```python
from build123d import *

# Parameters (mm, degrees)
SKETCH_1_R                = 20
SKETCH_1_R_2              = 11
EXTRUDE_1_DEPTH           = 60
EXTRUDE_2_DEPTH           = 30
SKETCH_4_R                = 11
EXTRUDE_3_DEPTH           = 5
SKETCH_8_R                = 11
CUT_EXTRUDE_1_DEPTH       = 100
FILLET_4_R                = 20
EXTRUDE_START             = -30
SKETCH_18_R               = 35
EXTRUDE_4_DEPTH           = 5
EXTRUDE_START_2           = -25
SKETCH_19_R               = 35
EXTRUDE_5_DEPTH           = 5
FILLET_5_R                = 10
CUT_EXTRUDE_9_DEPTH       = 388.169213652
CUT_EXTRUDE_9_DEPTH_BACK  = 388.169213652
SKETCH_21_R               = 2.6
CUT_EXTRUDE_10_DEPTH      = 407.881000043
CUT_EXTRUDE_10_DEPTH_BACK = 407.881000043
SKETCH_22_W               = 65
SKETCH_22_H               = 431.087956996
MOVE_FACE_1_BY            = 0.1


with BuildPart() as part:
    # 草图1 → 凸台-拉伸1 (new body)
    with BuildSketch(Plane.XY):
        Circle(SKETCH_1_R)
        Circle(SKETCH_1_R_2, mode=Mode.SUBTRACT)
    extrude(amount=EXTRUDE_1_DEPTH)

    # 草图2 → 凸台-拉伸2 (add, symmetric)
    with BuildSketch(Plane.XY.offset(30)):
        with BuildLine():
            Line((-14.142135624, 14.142135624), (-90, -61.715728753))
            Line((-90, -61.715728753), (-90, -320))
            Line((-90, -320), (-50, -320))
            Line((-50, -320), (-50, -78.284271247))
            Line((-50, -78.284271247), (14.142135624, -14.142135624))
            ThreePointArc((14.142135624, -14.142135624), (-14.142135624, -14.142135624), (-14.142135624, 14.142135624))
        make_face()
    extrude(amount=EXTRUDE_2_DEPTH, both=True)

    # 草图4 → 凸台-拉伸3 (add)
    with BuildSketch(Plane.XY.offset(60)):
        with BuildLine():
            Line((-90, -290), (-50, -290))
            Line((-50, -290), (-50, -350))
            ThreePointArc((-50, -350), (-70, -370), (-90, -350))
            Line((-90, -350), (-90, -290))
        make_face()
        with Locations((-70, -350)):
            Circle(SKETCH_4_R, mode=Mode.SUBTRACT)
    extrude_3 = extrude(amount=EXTRUDE_3_DEPTH)

    # 镜向1: 凸台-拉伸3 across plane
    add(extrude_3.mirror(Plane.XY.offset(30)))

    # 草图8 → 切除-拉伸1 (cut)
    with BuildSketch(Plane.XY.offset(60)):
        with Locations((-35.355339059, -35.355339059)):
            Circle(SKETCH_8_R)
    extrude(amount=-CUT_EXTRUDE_1_DEPTH, mode=Mode.SUBTRACT)

    # 圆角4
    fillet_4_edges = [part.edges().sort_by_distance(p)[0] for p in [
        (-50, -78.284271247, 30),
        (-90, -61.715728753, 30),
    ]]
    fillet(fillet_4_edges, radius=FILLET_4_R)

    # 草图18 → 凸台-拉伸4 (add)
    with BuildSketch(Plane.XY.offset(60).offset(EXTRUDE_START)):
        with BuildLine():
            ThreePointArc((15.487252676, -12.654841151), (14.833346688, -13.415357842), (14.142135624, -14.142135624))
            Line((14.142135624, -14.142135624), (-44.142135624, -72.426406871))
            ThreePointArc((-44.142135624, -72.426406871), (-48.47759065, -78.914873848), (-50, -86.568542495))
            Line((-50, -86.568542495), (-50, -128.513280962))
            Line((-50, -128.513280962), (20.291868618, -128.513280962))
            ThreePointArc((20.291868618, -128.513280962), (62.790327113, -100.116718851), (52.818780552, -49.986369028))
            Line((52.818780552, -49.986369028), (15.487252676, -12.654841151))
        make_face()
        with Locations((20.291868618, -82.513280962)):
            Circle(SKETCH_18_R, mode=Mode.SUBTRACT)
    extrude(amount=EXTRUDE_4_DEPTH)

    # 草图19 → 凸台-拉伸5 (add)
    with BuildSketch(Plane(origin=(0, 0, 0), x_dir=(-1, 0, 0), z_dir=(0, 0, -1)).offset(EXTRUDE_START_2)):
        with BuildLine():
            Line((50, -134.571348531), (50, -226.571348531))
            Line((50, -226.571348531), (-0.680255104, -226.571348531))
            ThreePointArc((-0.680255104, -226.571348531), (-46.680255104, -180.571348531), (-0.680255104, -134.571348531))
            Line((-0.680255104, -134.571348531), (50, -134.571348531))
        make_face()
        with Locations((-0.680255104, -180.571348531)):
            Circle(SKETCH_19_R, mode=Mode.SUBTRACT)
    extrude(amount=-EXTRUDE_5_DEPTH)

    # 圆角5
    # the kernel refuses this fillet: 10 mm, written as the material it adds along each edge
    with BuildSketch(Plane(origin=(-50, -226.571348531, 25), x_dir=(0, -1, 0), z_dir=(0, 0, 1)), Plane(origin=(-50, -128.513280962, 30), x_dir=(0, -1, 0), z_dir=(0, 0, 1))) as fillet_5_piece_1:
        with BuildLine():
            CenterArc((FILLET_5_R, FILLET_5_R), FILLET_5_R, 180, 90)
            Line((0, FILLET_5_R), (0, 0))
            Line((0, 0), (FILLET_5_R, 0))
        make_face()
    extrude(amount=5)

    # 草图21 → 切除-拉伸9 (cut, two sides: drawn at the far end of the back side and taken through both)
    with BuildSketch(Plane.XY.offset(65).offset(-CUT_EXTRUDE_9_DEPTH_BACK)):
        with Locations((-70, -75)):
            Circle(SKETCH_21_R)
        with Locations((-70, -250)):
            Circle(SKETCH_21_R)
        with Locations((-58, -300)):
            Circle(SKETCH_21_R)
        with Locations((-82, -300)):
            Circle(SKETCH_21_R)
    extrude(amount=CUT_EXTRUDE_9_DEPTH + CUT_EXTRUDE_9_DEPTH_BACK, mode=Mode.SUBTRACT)

    # 草图22 → 切除-拉伸10 (cut, two sides: drawn at the far end of the back side and taken through both)
    with BuildSketch(Plane.ZY.offset(90).offset(-CUT_EXTRUDE_10_DEPTH_BACK)):
        with Locations((32.5, -154.456021502)):
            Rectangle(SKETCH_22_W, SKETCH_22_H)
    extrude(amount=CUT_EXTRUDE_10_DEPTH + CUT_EXTRUDE_10_DEPTH_BACK, mode=Mode.SUBTRACT)

    # Move Face 1: a curved face moved inward by 0.1
    add(Solid.thicken(part.faces().sort_by_distance((-81, -350, -2.5))[0], -MOVE_FACE_1_BY), mode=Mode.SUBTRACT)


solid = part.part
```
Input: part model. Units: mm. Frame: model coordinates. Coordinates: 2 decimals unless noted, no trailing zeros. Loops run counter-clockwise (first coordinate to the right, second up) from the corner with the lowest first, then second, coordinate; pieces in that order, holes last. Notation, with made-up numbers: M 51,49 L 96,49 A28 cw 96,76 Z; hole C -28,57.5 d10. An arc over 180 degrees is marked long. Answer in a Markdown table with one row per item.
1. First-contact query: pin 1 (6 mm diameter, centred on x = -82, y = -300, fed in from -Z); pin 2 (2 mm diameter, centred on x = -78, z = -2, fed in from -Y) (3 decimals); pin 3 (1 mm diameter, centred on x = -76.5, z = -2, fed in from -Y). Flat tips, straight axial feed; report the tip coordinate or a pass-through.
Response:
| item | result |
|---|---|
| pin 1 | stops at z = -5 |
| pin 2 | stops at y = -368.735 |
| pin 3 | stops at y = -369.08 |
2. Section D-D, the plane y = -362. Output: boundary loops of the cut face in (x, z).
Response:
| item | result |
|---|---|
| outline | M -86,-5 L -54,-5 L -54,0 L -86,0 Z |
3. Section C-C, the plane x = -82. Output: boundary loops of the cut face in (y, z), then the cut area to 3 significant figures.
Response:
| item | result |
|---|---|
| outline | M -366,-5 L -302.6,-5 L -302.6,0 L -366,0 Z; M -297.4,-5 L -290,-5 L -290,0 L -297.4,0 Z |
| area | 354 mm2 |
4. Material intervals for line 1 (X direction, y = -300, z = -1.75); line 2 (Y direction, x = -70, z = -3.6); line 3 (Y direction, x = -67, z = -2.3), sorted ascending.
Response:
| item | result |
|---|---|
| line 1 | x = -90 to -84.6, -79.4 to -60.6, -55.4 to -50 |
| line 2 | y = -370 to -361.1, -338.9 to -290 |
| line 3 | y = -369.77 to -360.69, -339.31 to -290 |
5. Section B-B, the plane y = -300. Output: boundary loops of the cut face in (x, z), then the cut area to 3 significant figures.
Response:
| item | result |
|---|---|
| outline | M -90,-5 L -84.6,-5 L -84.6,0 L -90,0 Z; M -79.4,-5 L -60.6,-5 L -60.6,0 L -79.4,0 Z; M -55.4,-5 L -50,-5 L -50,0 L -55.4,0 Z |
| area | 148 mm2 |
6. Draft query along X for faces 1 (the cylindrical face through (-83.916, -298.243, -2.535)), 2 (the cylindrical face through (-70, -370, -2)), 3 (the flat face through (-70, -321, 0)). Return one class per face: pulls with the +X half, pulls with the -X half, needs draft (parallel to the pull), parting line crosses it, or undercut.
Response:
| item | result |
|---|---|
| face 1 | undercut |
| face 2 | parting line crosses it |
| face 3 | needs draft |
7. Section A-A, the plane x = -70. Output: boundary loops of the cut face in (y, z).
Response:
| item | result |
|---|---|
| outline | M -370,-5 L -361.1,-5 L -361.1,0 L -370,0 Z; M -338.9,-5 L -290,-5 L -290,0 L -338.9,0 Z |
